Autodesk Inventor part; units mm, degrees
ref_plane "YZ Plane" through (0, 0, 0) normal (1, 0, 0) x (0, 1, 0)
ref_plane "XZ Plane" through (0, 0, 0) normal (0, 1, 0) x (-1, 0, 0)
ref_plane "XY Plane" through (0, 0, 0) normal (0, 0, 1) x (1, 0, 0)
sketch "Sketch1" plane through (0, 0, 0) normal (0, 0, 1) x (1, 0, 0)
  line L0 (0, -8.1326) -> (0, 105.7239)
  line L1 (-30.6691, 0) -> (36.0366, 0)
  line L2 (0, 31.75) -> (0, 36.8263)
  arc A0 (0, 36.8263) -> (-0.8357, 43.3529) centre (-25.9044, 36.8263) ccw
  line L3 (-0.8357, 43.3529) -> (-6.8264, 66.3636)
  arc A1 (-7.531, 71.8662) -> (-6.8264, 66.3636) centre (14.3094, 71.8662) ccw
  line L4 (-7.531, 71.8662) -> (-7.531, 74.5808)
  arc A2 (-6.007, 76.1048) -> (-7.531, 74.5808) centre (-6.007, 74.5808) ccw
  line L5 (-6.007, 76.1048) -> (21.7425, 76.1048)
  line L6 (21.7425, 80.1688) -> (-6.007, 80.1688)
  arc A3 (-6.007, 80.1688) -> (-11.595, 74.5808) centre (-6.007, 74.5808) ccw
  line L7 (-11.595, 74.5808) -> (-11.595, 71.8662)
  arc A4 (-11.595, 71.8662) -> (-10.7593, 65.3396) centre (14.3094, 71.8662) ccw
  line L8 (-10.7593, 65.3396) -> (-4.7686, 42.329)
  arc A5 (-4.064, 36.8263) -> (-4.7686, 42.329) centre (-25.9044, 36.8263) ccw
  line L9 (-4.064, 36.8263) -> (-4.064, 31.75)
  line L10 (-4.064, 31.75) -> (0, 31.75)
  line L11 (21.7425, 80.1688) -> (21.7425, 76.1048)
  point P0 (0, 0)
  dimension "d0" = 33.3375
  dimension "d1" = 4.064
  dimension "d2" = 1.524
  dimension "d3" = 63.5
  dimension "d4" = 160.3375
revolve "Revolution1" add sketch "Sketch1" angle 360 about axis through (-10, 0, 0) along (1, 0, 0) contours L10 L9 A5 L8 A4 L7 A3 L6 L0 L5 A2 L4 A1 L3 A0 | L0 L6 L11 L5
properties part number "BrakeDrum"
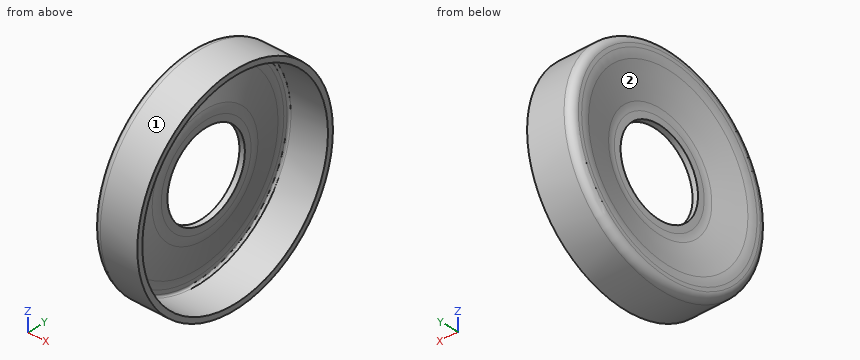
Input: part model. Units: mm. Frame: model coordinates. Face numbers are marked on the shaded views. Give positions to 0.01 mm unless a question says otherwise; leave off trailing zeros. Loops run counter-clockwise (first coordinate to the right, second up) from the corner with the lowest first, then second, coordinate; pieces in that order, holes last. Notation, with made-up numbers: M 86,49 L 140,49 A26 cw 140,76 Z; hole C -33.5,-4 d10. An arc over 180 degrees is marked long. Answer as CSV lines item,"result". Start each with the question number.
1. Section C-C on x = 18. Return loops of the section in (y, z).
2. Pull-direction query (Z, two-part tool) for the marked faces 1 and 2; classes: released by +Z, released by -Z, zero draft, split by the parting line, or undercut.
3. Line query: L1, parallel to Z at x = 13, y = 0; L2, parallel to Y at x = 4, z = 1; L3, parallel to Z at x = 10, y = 45. Output: solid intervals per line, ascending.
4. Pin query (flat end, axial travel): P1, Ø1, axis at x = 0.5, z = 62, coming from the -Y side; P2, Ø1, axis at x = -2, z = 51, coming from the -Y side; P3, Ø22, axis at y = 9.5, z = -18.5, coming from the +X side; P4, Ø22, axis at y = -10.5, z = 1.5, coming from the -X side. Return the tip coordinate at first contact, or that it passes through.
Computed values:
1,outline,"C 0,0 d160.34; hole C 0,0 d152.21"
2,face 1,"split by the parting line"
2,face 2,"undercut"
3,L1,"z = -80.17 to -76.1, 76.1 to 80.17"
3,L2,"y = -80.16 to -76.1, 76.1 to 80.16"
3,L3,"z = -66.35 to -61.38, 61.38 to 66.35"
4,P1,"stops at y = -51.43"
4,P2,"stops at y = -62.26"
4,P3,"stops at x = 0"
4,P4,"passes through"
